```python
from build123d import *

# Parameters (mm, degrees)
SKETCH1_W           = 96
SKETCH1_H           = 96
BOSS_EXTRUDE1_DEPTH = 15.494
SKETCH2_W           = 127
SKETCH2_H           = 111.5
BOSS_EXTRUDE2_DEPTH = 1.27
SHELL1_START        = -46.73
SHELL1_OUTLINE_W    = 94.73
SHELL1_OUTLINE_H    = 14.224
SHELL1_DEPTH        = 93.46


# Read off the part's stored shape, not the designer's step: Shell1
with BuildPart() as part:
    # Sketch1 → Boss-Extrude1 (new body)
    with BuildSketch(Plane.XY):
        Rectangle(SKETCH1_W, SKETCH1_H)
    extrude(amount=BOSS_EXTRUDE1_DEPTH)

    # Sketch2 → Boss-Extrude2 (add)
    with BuildSketch(Plane.XY.offset(15.494)):
        with Locations((0, -7.75)):
            Rectangle(SKETCH2_W, SKETCH2_H)
    extrude(amount=-BOSS_EXTRUDE2_DEPTH)

    # Shell1 outline → Shell1 (cut)
    with BuildSketch(Plane.YZ.offset(SHELL1_START)):
        with Locations((0.635, 8.382)):
            Rectangle(SHELL1_OUTLINE_W, SHELL1_OUTLINE_H)
    extrude(amount=SHELL1_DEPTH, mode=Mode.SUBTRACT)


solid = part.part
```
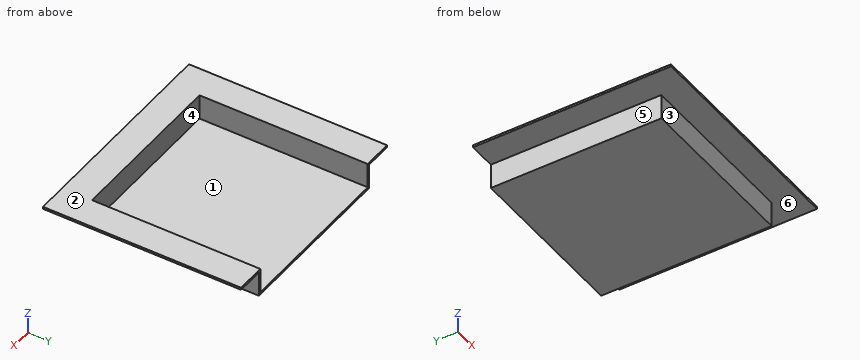
Geometry: final body of the model. Coordinates: model frame, mm. Face numbers are marked on the shaded views. A direction names the side the tool comes from. Coordinates: 2 decimals unless noted, no trailing zeros. Order: outer loops, then holes, each group sorted by start corner. A loop starts at its lowest first (then second) coordinate and runs counter-clockwise, first axis right, second up. Notation, with made-up numbers: M -2.75,70.25 L 3.25,70.25 A17 cw 3.25,84.25 Z; hole C 44,-4.5 d7. An arc over 180 degrees is marked long. Answer in a Markdown table with one row per item. Add a question column.
Q1. Section query A-A on z = 10.25. Return the cut outline in (x, y), and give its area (3 significant figures).
Q2. Mould query, pull axis X, two halves, no side actions, for the marked faces 4, 5 and 6. Classes: released by +X, released by -X, zero draft, split by the parting line, or undercut.
Q3. Section query C-C on y = -15. Return the cut outline in (x, z).
Q4. Contact query for flat-ended pins moving along their axis: P1, Ø4.5, axis at x = -5, z = 6.5, coming from the -Y side; P2, Ø8, axis at y = -21, z = 6, coming from the -X side; P3, Ø1, axis at x = -16.5, z = 3, coming from the +Y side; P4, Ø1, axis at x = -49.5, z = 8, coming from the -Y side. Output: stop coordinate, or through.
Q5. Reachability of the marked faces 1, 2 and 3 from +Z, -Z, +X, -X, +Y, -Y: full face, straight path, thin tool, end or side. Return the list, or none.
Q6. Line query: L1, parallel to X at y = -39.5, z = 4.5; L2, parallel to Z at x = 2, y = 23.5; L3, parallel to Y at x = 38.5, z = 3.25. Output: solid intervals per line, ascending.
Q7. Section query B-B on x = -21.5. Return the cut outline in (y, z).
Completed:
| question | item | result |
|---|---|---|
| 1 | outline | M -48,-48 L 48,-48 L 48,48 L 46.73,48 L 46.73,-46.73 L -46.73,-46.73 L -46.73,48 L -48,48 Z |
| 1 | area | 363 mm2 |
| 2 | face 4 | undercut |
| 2 | face 5 | released by -X |
| 2 | face 6 | zero draft |
| 3 | outline | M -63.5,14.22 L -48,14.22 L -48,0 L 48,0 L 48,14.22 L 63.5,14.22 L 63.5,15.49 L 46.73,15.49 L 46.73,1.27 L -46.73,1.27 L -46.73,15.49 L -63.5,15.49 Z |
| 4 | P1 | stops at y = -48 |
| 4 | P2 | stops at x = -48 |
| 4 | P3 | stops at y = -46.73 |
| 4 | P4 | passes through |
| 5 | face 1 | +Z, +Y |
| 5 | face 2 | +Z, +X, -X, +Y, -Y |
| 5 | face 3 | -Z, +X, -X, -Y |
| 6 | L1 | x = -48 to -46.73, 46.73 to 48 |
| 6 | L2 | z = 0 to 1.27 |
| 6 | L3 | y = -48 to -46.73 |
| 7 | outline | M -63.5,14.22 L -48,14.22 L -48,0 L 48,0 L 48,1.27 L -46.73,1.27 L -46.73,15.49 L -63.5,15.49 Z |
